Can you work these out from the drawing? Everything is in mm from the part's minimum corner. Coordinates: 2 decimals unless noted, no trailing zeros. Order: outer loops, then holes, each group sorted by start corner. A loop starts at its lowest first (then second) coordinate and runs counter-clockwise, first axis right, second up. Notation, with made-up numbers: (64, 86) -> (101, 86) arc R21 ccw to (101, 122) -> close; hole circle Ø10 at (73, -3.5). An arc over 180 degrees is marked (long way). Return JSON: item names as keys, results as strings. Group by question number.
1) If we section it at C-C, the plane z = 6.25: State how many separate pieces and enclosed holes the cut face has, then the cut area to 3 significant figures.
2) If we section it at A-A, the plane y = 50: Please give me the cut outline in (x, z).
3) If I drill on probe 1 along Y at (x, z) = (140, 5); probe 2 along Y at (x, z) = (165, 4.5); probe 3 along X at (y, z) = (50, 2.5), over which ranges is the centre line in solid material (lowest first)? Write a range as from..to.
4) If we section it at B-B, the plane x = 30: Please give me the cut outline in (y, z).
5) If we section it at D-D, the plane y = 5: Please give me the cut outline in (x, z).
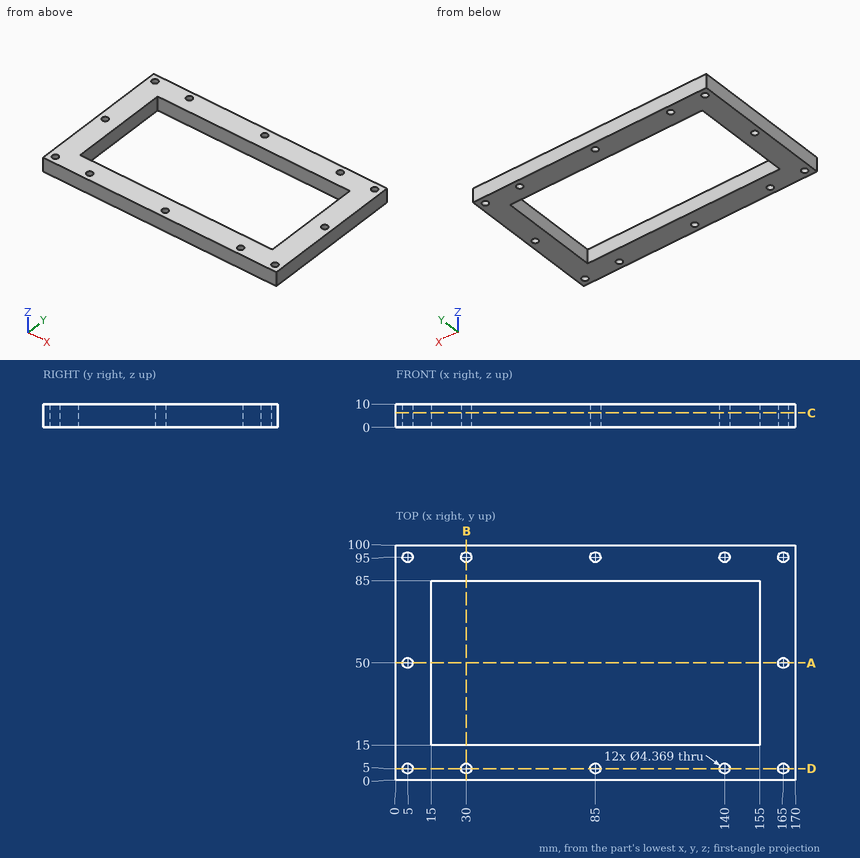
Result sheet:
{
 "1": {"separate pieces": "1", "enclosed holes": "13", "area": "7,020 mm2"},
 "2": {"outline": "(0, 0) -> (2.82, 0) -> (2.82, 10) -> (0, 10) -> close; (7.18, 0) -> (15, 0) -> (15, 10) -> (7.18, 10) -> close; (155, 0) -> (162.82, 0) -> (162.82, 10) -> (155, 10) -> close; (167.18, 0) -> (170, 0) -> (170, 10) -> (167.18, 10) -> close"},
 "3": {"probe 1": "y = 0..2.82, 7.18..15, 85..92.82, 97.18..100", "probe 2": "y = 0..2.82, 7.18..47.82, 52.18..92.82, 97.18..100", "probe 3": "x = 0..2.82, 7.18..15, 155..162.82, 167.18..170"},
 "4": {"outline": "(0, 0) -> (2.82, 0) -> (2.82, 10) -> (0, 10) -> close; (7.18, 0) -> (15, 0) -> (15, 10) -> (7.18, 10) -> close; (85, 0) -> (92.82, 0) -> (92.82, 10) -> (85, 10) -> close; (97.18, 0) -> (100, 0) -> (100, 10) -> (97.18, 10) -> close"},
 "5": {"outline": "(0, 0) -> (2.82, 0) -> (2.82, 10) -> (0, 10) -> close; (7.18, 0) -> (27.82, 0) -> (27.82, 10) -> (7.18, 10) -> close; (32.18, 0) -> (82.82, 0) -> (82.82, 10) -> (32.18, 10) -> close; (87.18, 0) -> (137.82, 0) -> (137.82, 10) -> (87.18, 10) -> close; (142.18, 0) -> (162.82, 0) -> (162.82, 10) -> (142.18, 10) -> close; (167.18, 0) -> (170, 0) -> (170, 10) -> (167.18, 10) -> close"}
}
